```python
from build123d import *

# Parameters (mm, degrees)
BOSS_EXTRUDE1_DEPTH = 1.75
SCALE1_SCALE        = 25.4


with BuildPart() as part:
    # Sketch1 → Boss-Extrude1 (new body)
    with BuildSketch(Plane.XY):
        with BuildLine():
            Line((0, 12), (0, 0))
            Line((0, 0), (8.625, 0))
            Line((8.625, 0), (8.625, 12))
            Line((8.625, 12), (6.8125, 12))
            Line((6.8125, 12), (6.8125, 6))
            ThreePointArc((6.8125, 6), (4.3125, 3.5), (1.8125, 6))
            Line((1.8125, 6), (1.8125, 12))
            Line((1.8125, 12), (0, 12))
        make_face()
    extrude(amount=BOSS_EXTRUDE1_DEPTH)


with BuildPart() as part_1:
    # Scale1: scaled about (4.3125, 4.750311237, 0.875)
    add(part.part.scale(SCALE1_SCALE).moved(Location((-105.225, -115.907594183, -21.35))))


solid = part_1.part
```
Read the model definition and answer for the solid it produces. Units are mm, in the model's axes. A direction names the side the tool comes from. Coordinates: 2 decimals unless noted, no trailing zeros. Write each loop counter-clockwise with the first axis right and the second up, starting at its lowest first coordinate (ties: lowest second). Pieces come first, ordered by that corner, then holes. Notation, with made-up numbers: (43.5, 74) -> (51.5, 74) arc R24 ccw to (51.5, 87) -> close; hole circle Ø10 at (-17, -32.5). An arc over 180 degrees is marked (long way). Return JSON: item names as keys, results as strings.
1. Determine the mould class of faces 1 (the face through (3, -115.908, 1)), 2 (the face through (5.709, -26.992, 0.564)), 3 (the face through (113.85, 34, 1)), 4 (the face through (-105.225, 39, 1)) for opening direction X: pulls with the +X half, pulls with the -X half, needs draft (parallel to the pull), parting line crosses it, or undercut.
Found:
{"face 1": "needs draft", "face 2": "undercut", "face 3": "pulls with the +X half", "face 4": "pulls with the -X half"}
2. A cutting plane is placed at C-C (x = -50.5). Determine the outline of the cut face in (y, z).
Found:
{"outline": "(-115.91, -21.35) -> (4.43, -21.35) -> (4.43, 23.1) -> (-115.91, 23.1) -> close"}
3. A tool of negligible diameter and unlimited length cuts with its end or side. For faces 5 (the face through (3, -29, -21.35)), 6 (the face through (67.812, 114, 1)), from which of +Z, -Z, +X, -X, +Y, -Y can it reach the whole face along a straight path? Write none if from no direction.
Found:
{"face 5": "-Z, +X, -X, +Y, -Y", "face 6": "+Z, -Z, +Y"}
4. This flat-tipped pin is pushed along its axis until it touches: P1, Ø2, axis at x = -22.5, z = 11.5, coming from the +Y side. Where does it stop, or does it pass through?
Found:
{"P1": "y = -20.59"}
5. Find the intervals of material crossed by line 1 along X through (y, z) = (-20.5, -4) (3 decimals); line 2 along Y through (x, z) = (9, 6.5); line 3 along Y through (x, z) = (-21, 4.5), in increasing order. Write a range as from..to.
Found:
{"line 1": "-105.225..-23.69, 32.315..113.85", "line 2": "-115.91..-26.83", "line 3": "-115.91..-21.74"}
